Input: part model. Units: mm. Frame: model coordinates. Coordinates: 2 decimals unless noted, no trailing zeros. Write each loop counter-clockwise with the first axis right and the second up, starting at its lowest first coordinate (ties: lowest second). Pieces come first, ordered by that corner, then holes. Notation, with made-up numbers: M 71.5,-12 L 100.5,-12 A13 ccw 100.5,-5 Z; hole C 89.25,88 d9. An arc over 180 degrees is marked long. Answer as a JSON object with one key per item and string values. Group by question number.
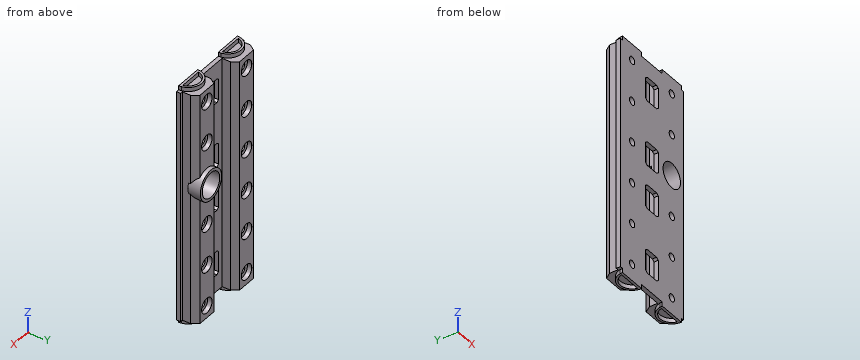
from build123d import *

# Parameters (mm, degrees)
BOSS_EXTRUDE1_DEPTH                         = 280
BOSS_EXTRUDE3_DEPTH                         = 5
MIRROR2_COPY_1_DEPTH                        = 5
CBORE_SLOT_FOR_M8_HEX_HEAD_BOLT1_AT_2_COUNT = 2
CBORE_SLOT_FOR_M8_HEX_HEAD_BOLT1_AT_2_PITCH = 50
CBORE_SLOT_FOR_M8_HEX_HEAD_BOLT1_AT_3_COUNT = 2
CBORE_SLOT_FOR_M8_HEX_HEAD_BOLT1_AT_3_PITCH = 100
CBORE_SLOT_FOR_M8_HEX_HEAD_BOLT1_AT_4_COUNT = 2
CBORE_SLOT_FOR_M8_HEX_HEAD_BOLT1_AT_4_PITCH = 150
CBORE_SLOT_FOR_M8_HEX_HEAD_BOLT1_AT_5_COUNT = 2
CBORE_SLOT_FOR_M8_HEX_HEAD_BOLT1_AT_5_PITCH = 200
CBORE_SLOT_FOR_M8_HEX_HEAD_BOLT1_AT_6_COUNT = 2
CBORE_SLOT_FOR_M8_HEX_HEAD_BOLT1_AT_6_PITCH = 250
BOSS_EXTRUDE4_DEPTH                         = 5
BOSS_EXTRUDE4_DEPTH_BACK                    = 10
SKETCH12_R                                  = 18.373536693
SKETCH14_R                                  = 15
CUT_EXTRUDE1_DEPTH                          = 28
CUT_EXTRUDE2_DEPTH                          = 294.662080045


with BuildPart() as part:
    # Sketch4 → Boss-Extrude1 (new body)
    with BuildSketch(Plane.XY):
        Polygon((-41.702855028, 2.5), (-38.702855028, 2.5), (-38.702855028, 12.5), (-33.495143371, 20), (-9.495143371, 20), (-4.287431713, 12.5), (-4.287431713, 2.5), (-1.287431713, 2.5), (26.712568287, 2.5), (29.712568287, 2.5), (29.712568287, 12.5), (34.920279944, 20), (58.920279944, 20), (64.127991602, 12.5), (64.127991602, 2.5), (67.127991602, 2.5), (67.127991602, -2.5), (26.712568287, -2.5), (-1.287431713, -2.5), (-41.702855028, -2.5), align=None)
    extrude(amount=-BOSS_EXTRUDE1_DEPTH)

    # Sketch5 → Boss-Extrude3 (add)
    with BuildSketch(Plane.XY):
        with BuildLine():
            ThreePointArc((-5.267870643, 0.487577586), (-21.495143371, 14), (-37.722416098, 0.487577586))
            Line((-37.722416098, 0.487577586), (-35.17265704, 0.487577586))
            ThreePointArc((-35.17265704, 0.487577586), (-21.495143371, 11.5), (-7.817629702, 0.487577586))
            Line((-7.817629702, 0.487577586), (-5.267870643, 0.487577586))
        make_face()
        Polygon((-37.722416098, 0.487577586), (-37.995143371, -2.5), (-4.995143371, -2.5), (-5.267870643, 0.487577586), (-7.817629702, 0.487577586), (-35.17265704, 0.487577586), align=None)
    boss_extrude3 = extrude(amount=BOSS_EXTRUDE3_DEPTH)

    # Mirror1: Boss-Extrude3 across plane
    add(boss_extrude3.mirror(Plane.ZY.offset(-12.712568287)))

    # Mirror2: Boss-Extrude3 across plane
    add(boss_extrude3.mirror(Plane.XY.offset(-140)))

    # Mirror2 copy 1 sketch → Mirror2 copy 1 (add)
    with BuildSketch(Plane(origin=(25.425136574, 0, -280), x_dir=(-1, 0, 0), z_dir=(0, 0, -1))):
        with BuildLine():
            ThreePointArc((-5.267870643, 0.487577586), (-21.495143371, 14), (-37.722416098, 0.487577586))
            Line((-37.722416098, 0.487577586), (-35.17265704, 0.487577586))
            ThreePointArc((-35.17265704, 0.487577586), (-21.495143371, 11.5), (-7.817629702, 0.487577586))
            Line((-7.817629702, 0.487577586), (-5.267870643, 0.487577586))
        make_face()
        Polygon((-37.722416098, 0.487577586), (-37.995143371, -2.5), (-4.995143371, -2.5), (-5.267870643, 0.487577586), (-7.817629702, 0.487577586), (-35.17265704, 0.487577586), align=None)
    extrude(amount=MIRROR2_COPY_1_DEPTH)

    # Sketch10 → CBORE SLOT for M8 Hex Head Bolt1 (revolve, cut)
    with BuildSketch(Plane(origin=(46.920279944, 20, -265), x_dir=(0, 0, 1), z_dir=(1, 0, 0))):
        Polygon((0, 0), (0, 34.543872786), (4.5, 31.84), (4.5, 5.3), (9.0055, 5.3), (9.0055, 0.025), (9.0305, 0), align=None)
    cbore_slot_for_m8_hex_head_bolt1 = revolve(axis=Axis((46.920279944, 26.35, -265), (0, -1, 0)), mode=Mode.SUBTRACT)

    # CBORE SLOT for M8 Hex Head Bolt1 at 2: CBORE SLOT for M8 Hex Head Bolt1 ×2
    with Locations(*[(0, 0, i * CBORE_SLOT_FOR_M8_HEX_HEAD_BOLT1_AT_2_PITCH) for i in range(1, CBORE_SLOT_FOR_M8_HEX_HEAD_BOLT1_AT_2_COUNT)]):
        add(cbore_slot_for_m8_hex_head_bolt1, mode=Mode.SUBTRACT)

    # CBORE SLOT for M8 Hex Head Bolt1 at 3: CBORE SLOT for M8 Hex Head Bolt1 ×2
    with Locations(*[(0, 0, i * CBORE_SLOT_FOR_M8_HEX_HEAD_BOLT1_AT_3_PITCH) for i in range(1, CBORE_SLOT_FOR_M8_HEX_HEAD_BOLT1_AT_3_COUNT)]):
        add(cbore_slot_for_m8_hex_head_bolt1, mode=Mode.SUBTRACT)

    # CBORE SLOT for M8 Hex Head Bolt1 at 4: CBORE SLOT for M8 Hex Head Bolt1 ×2
    with Locations(*[(0, 0, i * CBORE_SLOT_FOR_M8_HEX_HEAD_BOLT1_AT_4_PITCH) for i in range(1, CBORE_SLOT_FOR_M8_HEX_HEAD_BOLT1_AT_4_COUNT)]):
        add(cbore_slot_for_m8_hex_head_bolt1, mode=Mode.SUBTRACT)

    # CBORE SLOT for M8 Hex Head Bolt1 at 5: CBORE SLOT for M8 Hex Head Bolt1 ×2
    with Locations(*[(0, 0, i * CBORE_SLOT_FOR_M8_HEX_HEAD_BOLT1_AT_5_PITCH) for i in range(1, CBORE_SLOT_FOR_M8_HEX_HEAD_BOLT1_AT_5_COUNT)]):
        add(cbore_slot_for_m8_hex_head_bolt1, mode=Mode.SUBTRACT)

    # CBORE SLOT for M8 Hex Head Bolt1 at 6: CBORE SLOT for M8 Hex Head Bolt1 ×2
    with Locations(*[(0, 0, i * CBORE_SLOT_FOR_M8_HEX_HEAD_BOLT1_AT_6_PITCH) for i in range(1, CBORE_SLOT_FOR_M8_HEX_HEAD_BOLT1_AT_6_COUNT)]):
        add(cbore_slot_for_m8_hex_head_bolt1, mode=Mode.SUBTRACT)

    # Mirror3: CBORE SLOT for M8 Hex Head Bolt1 across plane
    add(cbore_slot_for_m8_hex_head_bolt1.mirror(Plane.ZY.offset(-12.712568287)), mode=Mode.SUBTRACT)

    # Mirror3 copy 1 sketch → Mirror3 copy 1 (revolve, cut)
    with BuildSketch(Plane(origin=(-21.495143371, 20, -215), x_dir=(0, 0, 1), z_dir=(-1, 0, 0))):
        Polygon((0, 0), (0, -34.543872786), (4.5, -31.84), (4.5, -5.3), (9.0055, -5.3), (9.0055, -0.025), (9.0305, 0), align=None)
    revolve(axis=Axis((-21.495143371, 26.35, -215), (0, 1, 0)), mode=Mode.SUBTRACT)

    # Mirror3 copy 2 sketch → Mirror3 copy 2 (revolve, cut)
    with BuildSketch(Plane(origin=(-21.495143371, 20, -165), x_dir=(0, 0, 1), z_dir=(-1, 0, 0))):
        Polygon((0, 0), (0, -34.543872786), (4.5, -31.84), (4.5, -5.3), (9.0055, -5.3), (9.0055, -0.025), (9.0305, 0), align=None)
    revolve(axis=Axis((-21.495143371, 26.35, -165), (0, 1, 0)), mode=Mode.SUBTRACT)

    # Mirror3 copy 3 sketch → Mirror3 copy 3 (revolve, cut)
    with BuildSketch(Plane(origin=(-21.495143371, 20, -115), x_dir=(0, 0, 1), z_dir=(-1, 0, 0))):
        Polygon((0, 0), (0, -34.543872786), (4.5, -31.84), (4.5, -5.3), (9.0055, -5.3), (9.0055, -0.025), (9.0305, 0), align=None)
    revolve(axis=Axis((-21.495143371, 26.35, -115), (0, 1, 0)), mode=Mode.SUBTRACT)

    # Mirror3 copy 4 sketch → Mirror3 copy 4 (revolve, cut)
    with BuildSketch(Plane(origin=(-21.495143371, 20, -65), x_dir=(0, 0, 1), z_dir=(-1, 0, 0))):
        Polygon((0, 0), (0, -34.543872786), (4.5, -31.84), (4.5, -5.3), (9.0055, -5.3), (9.0055, -0.025), (9.0305, 0), align=None)
    revolve(axis=Axis((-21.495143371, 26.35, -65), (0, 1, 0)), mode=Mode.SUBTRACT)

    # Mirror3 copy 5 sketch → Mirror3 copy 5 (revolve, cut)
    with BuildSketch(Plane(origin=(-21.495143371, 20, -15), x_dir=(0, 0, 1), z_dir=(-1, 0, 0))):
        Polygon((0, 0), (0, -34.543872786), (4.5, -31.84), (4.5, -5.3), (9.0055, -5.3), (9.0055, -0.025), (9.0305, 0), align=None)
    revolve(axis=Axis((-21.495143371, 26.35, -15), (0, 1, 0)), mode=Mode.SUBTRACT)

    # Sketch12 → Boss-Extrude4 (add, two sides: drawn at the far end of the back side and taken through both)
    with BuildSketch(Plane(origin=(0, 20, 0), x_dir=(1, 0, 0), z_dir=(0, 1, 0)).offset(-BOSS_EXTRUDE4_DEPTH_BACK)):
        with Locations(Location((46.920279944, 115, 0), (0, 0, 270))):
            Circle(SKETCH12_R)
    extrude(amount=BOSS_EXTRUDE4_DEPTH + BOSS_EXTRUDE4_DEPTH_BACK)

    # Sketch14 → Cut-Extrude1 (cut)
    with BuildSketch(Plane(origin=(0, 25, 0), x_dir=(1, 0, 0), z_dir=(0, 1, 0))):
        with Locations(Location((46.920279944, 115, 0), (0, 0, 270))):
            Circle(SKETCH14_R)
    extrude(amount=-CUT_EXTRUDE1_DEPTH, mode=Mode.SUBTRACT)

    # Sketch16 → Cut-Extrude2 (cut, through all)
    with BuildSketch(Plane(origin=(0, 2.5, 0), x_dir=(1, 0, 0), z_dir=(0, 1, 0))):
        Polygon((20.712568287, 20), (4.712568287, 20), (1.802568287, 22), (1.802568287, 47), (4.712568287, 49), (20.712568287, 49), (23.622568287, 47), (23.622568287, 22), align=None)
        Polygon((23.622568287, 101), (20.712568287, 99), (4.712568287, 99), (1.802568287, 101), (1.802568287, 126), (4.712568287, 128), (20.712568287, 128), (23.622568287, 126), align=None)
    cut_extrude2 = extrude(amount=-CUT_EXTRUDE2_DEPTH, mode=Mode.SUBTRACT)

    # Mirror4: Cut-Extrude2 across plane
    add(cut_extrude2.mirror(Plane.XY.offset(-140)), mode=Mode.SUBTRACT)


solid = part.part
Q1. Section B-B, the plane z = -115. State how many separate pieces and enclosed holes the cut face has, and give its area (3 significant figures).
Q2. Pin query (flat end, axial travel): pin 1 Ø5.5 at (x, z) = (47.5, -213) entering from +Y; pin 2 Ø2.5 at (x, y) = (9.5, 0.5) entering from +Z; pin 3 Ø12 at (y, z) = (14, -49.5) entering from +X. Return the tip coordinate at first contact, or that it passes through.
Q3. Section A-A, the plane z = -243. Return the cut outline in (x, y), and give its area (3 significant figures).
Q4. Line query: line 1 (X direction, y = 10.75, z = -65); line 2 (Z direction, x = 5, y = -1); line 3 (X direction, y = 9, z = -181.5). Output: solid intervals per line, ascending. Write a range as from..to.
Filled in:
{
 "1": {"separate pieces": "4", "enclosed holes": "0", "area": "732 mm^2"},
 "2": {"pin 1": "y = 14.7", "pin 2": "z = 0", "pin 3": "x = 64.13"},
 "3": {"outline": "M -41.7,-2.5 L 1.8,-2.5 L 1.8,2.5 L -4.29,2.5 L -4.29,12.5 L -9.5,20 L -33.5,20 L -38.7,12.5 L -38.7,2.5 L -41.7,2.5 Z; M 23.62,-2.5 L 67.13,-2.5 L 67.13,2.5 L 64.13,2.5 L 64.13,12.5 L 58.92,20 L 34.92,20 L 29.71,12.5 L 29.71,2.5 L 23.62,2.5 Z", "area": "1,560 mm^2"},
 "4": {"line 1": "-38.7..-26, -17..-4.29, 29.71..42.42, 51.42..64.13", "line 2": "-280..-260, -231..-181, -152..-128, -99..-49, -20..0", "line 3": "-38.7..-4.29, 29.71..64.13"}
}
